Geometry check sheet. Reference: the model listing, model coordinates, mm. A direction names the side the tool comes from. Coordinates: 2 decimals unless noted, no trailing zeros. Loops run counter-clockwise (first coordinate to the right, second up) from the corner with the lowest first, then second, coordinate; pieces in that order, holes last. Notation, with made-up numbers: M 87,57.5 L 110,57.5 A15 cw 110,71.5 Z; hole C 69.5,15 d1. An arc over 180 degrees is marked long. Use CSV: the item, a comma, the result in double quotes.
```python
from build123d import *

# Parameters (mm, degrees)
F0_W     = 38.1
F0_H     = 38.1
F1_DEPTH = 50.8
F2_T     = -2.54
F3_DEPTH = 25.4
F4_T     = -2.54


# Not quite as in the source:
# - a shell that OpenCascade refuses in one call is made with other operations: the cavity is built on its own and cut out


with BuildPart() as f1:
    # F0 (on Top) → F1 (new body)
    with BuildSketch(Plane.XY):
        Rectangle(F0_W, F0_H)
    extrude(amount=F1_DEPTH)

    # F2
    f2_openings = [f1.faces().sort_by_distance(p)[0] for p in [
        (0, 0, 50.8),
    ]]
    offset(amount=F2_T, openings=f2_openings)

    # F0 (on Top) → F3 (join)
    with BuildSketch(Plane.XY):
        with Locations((38.1, 0)):
            Rectangle(F0_W, F0_H)
    extrude(amount=F3_DEPTH)

    # F4: a shell. OpenCascade refuses it in one call, so the cavity is built on its own and cut out:
    # the body offset inwards by the wall thickness, plus a prism from it out through each open face.
    f4_core = offset(f1.part, amount=F4_T, kind=Kind.INTERSECTION, mode=Mode.PRIVATE)
    f4_exits = [f4_core.faces().sort_by_distance(p)[0] for p in [
        (36.83, 0, 22.86),
    ]]
    add(f4_core, mode=Mode.SUBTRACT)
    extrude(f4_exits, amount=-F4_T, mode=Mode.SUBTRACT)


solid = f1.part
```
1. Section check B-B, the plane z = 45. Record the cut outline in (x, y).
The answers:
outline,"M -19.05,-19.05 L 19.05,-19.05 L 19.05,19.05 L -19.05,19.05 Z; hole M -16.51,-16.51 L 16.51,-16.51 L 16.51,16.51 L -16.51,16.51 Z"
2. Section check C-C, the plane x = 41. Record the cut outline in (y, z).
The answers:
outline,"M -19.05,0 L 19.05,0 L 19.05,25.4 L 16.51,25.4 L 16.51,2.54 L -16.51,2.54 L -16.51,25.4 L -19.05,25.4 Z"
3. Release check for a two-part mould opening along Y. For faces 4 (the flat face through (10, 19.05, 19)), 5 (the flat face through (10, -19.05, 19)), 6 (the flat face through (0, 16.51, 26)), 7 (the flat face through (19, 0, 0)) record: +Y half, -Y half, draft (parallel to the pull), parting line (faces both ways), or undercut.
The answers:
face 4,"+Y half"
face 5,"-Y half"
face 6,"undercut"
face 7,"draft"
4. Gauge pin test, flat ends, axial feed: P1, Ø2, axis at x = -2, y = -12.5, coming from the +Z side; P2, Ø5, axis at y = -7, z = 30, coming from the +X side. Record the tip position at first contact, or that the pin passes through.
The answers:
P1,"z = 2.54"
P2,"x = 19.05"
5. Thickness scan on line 1 (X direction, y = 8, z = 13.5); line 2 (Y direction, x = 39.5, z = 10.5). Record the ranges inside material, lowest first. Write a range as [from, to].
The answers:
line 1,"[-19.05, -16.51], [16.51, 19.05], [54.61, 57.15]"
line 2,"[-19.05, -16.51], [16.51, 19.05]"
6. Section check D-D, the plane y = -12. Record the cut outline in (x, z), plus the area to 3 significant figures.
The answers:
outline,"M -19.05,0 L 57.15,0 L 57.15,25.4 L 54.61,25.4 L 54.61,2.54 L 19.05,2.54 L 19.05,50.8 L 16.51,50.8 L 16.51,2.54 L -16.51,2.54 L -16.51,50.8 L -19.05,50.8 Z"
area,"497 mm^2"
7. Set-up check for faces 1 (the flat face through (19.05, 0, 26)), 2 (the flat face through (55, -3, 25.4)), 3 (the flat face through (-19.05, 0, 25)): record each of +Z, -Z, +X, -X, +Y, -Y from which the full face is reachable in a straight line by a thin tool's end or side.
The answers:
face 1,"+Z"
face 2,"+Z, +X, +Y, -Y"
face 3,"+Z, -Z, -X, +Y, -Y"
8. Section check A-A, the plane z = 6. Record the cut outline in (x, y), plus the area to 3 significant figures.
The answers:
outline,"M -19.05,-19.05 L 57.15,-19.05 L 57.15,19.05 L -19.05,19.05 Z; hole M -16.51,-16.51 L 16.51,-16.51 L 16.51,16.51 L -16.51,16.51 Z; hole M 19.05,-16.51 L 54.61,-16.51 L 54.61,16.51 L 19.05,16.51 Z"
area,"639 mm^2"
